```python
from build123d import *

# Parameters (mm, degrees)
ESQUISSE1_W        = 94
ESQUISSE1_H        = 61
ESQUISSE1_R        = 1.75
BOSS_EXTRU_1_DEPTH = 1.6
ESQUISSE2_W        = 50
ESQUISSE2_H        = 25
BOSS_EXTRU_2_DEPTH = 18
ESQUISSE3_W        = 9
ESQUISSE3_H        = 14
BOSS_EXTRU_3_DEPTH = 11


with BuildPart() as part:
    # Esquisse1 → Boss.-Extru.1 (new body)
    with BuildSketch(Plane.XY):
        Rectangle(ESQUISSE1_W, ESQUISSE1_H)
        with Locations((-42, 25.5)):
            Circle(ESQUISSE1_R, mode=Mode.SUBTRACT)
        with Locations((42, 25.5)):
            Circle(ESQUISSE1_R, mode=Mode.SUBTRACT)
        with Locations((42, -25.5)):
            Circle(ESQUISSE1_R, mode=Mode.SUBTRACT)
        with Locations((-42, -25.5)):
            Circle(ESQUISSE1_R, mode=Mode.SUBTRACT)
    extrude(amount=BOSS_EXTRU_1_DEPTH)

    # Esquisse2 → Boss.-Extru.2 (add)
    with BuildSketch(Plane.XY.offset(1.6)):
        Rectangle(ESQUISSE2_W, ESQUISSE2_H)
    extrude(amount=BOSS_EXTRU_2_DEPTH)

    # Esquisse3 → Boss.-Extru.3 (add)
    with BuildSketch(Plane.XY.offset(1.6)):
        with Locations((-31.5, -23.5)):
            Rectangle(ESQUISSE3_W, ESQUISSE3_H)
    extrude(amount=BOSS_EXTRU_3_DEPTH)


solid = part.part
```
Design review of the part built by this model. Coordinates are the model's own, in mm. A direction names the side the tool comes from. Give positions to 0.01 mm unless a question says otherwise; leave off trailing zeros. Write each loop counter-clockwise with the first axis right and the second up, starting at its lowest first coordinate (ties: lowest second). Pieces come first, ordered by that corner, then holes. Notation, with made-up numbers: (0.25, 89) -> (14.25, 89) arc R7 ccw to (14.25, 96) -> close; hole circle Ø9 at (65, 44.5). An arc over 180 degrees is marked (long way). Answer in a Markdown table with one row per item.
(1) Consider section A-A (x = 42). State the section outline as (y, z) points.
Results:
| item | result |
|---|---|
| outline | (-30.5, 0) -> (-27.25, 0) -> (-27.25, 1.6) -> (-30.5, 1.6) -> close; (-23.75, 0) -> (23.75, 0) -> (23.75, 1.6) -> (-23.75, 1.6) -> close; (27.25, 0) -> (30.5, 0) -> (30.5, 1.6) -> (27.25, 1.6) -> close |
(2) Consider section C-C (y = -25.5). State the section outline as (x, z) points.
Results:
| item | result |
|---|---|
| outline | (-47, 0) -> (-43.75, 0) -> (-43.75, 1.6) -> (-47, 1.6) -> close; (-40.25, 0) -> (40.25, 0) -> (40.25, 1.6) -> (-27, 1.6) -> (-27, 12.6) -> (-36, 12.6) -> (-36, 1.6) -> (-40.25, 1.6) -> close; (43.75, 0) -> (47, 0) -> (47, 1.6) -> (43.75, 1.6) -> close |
(3) For faces 4 (the flat face through (-25, 0, 10)), 5 (the flat face through (25, 0, 10)), 6 (the flat face through (0, 12.5, 10)), list the 3-axis set-ups (+Z, -Z, +X, -X, +Y, -Y) from which the entire face can be reached by the end or side of a thin tool; tool diameter is ignored.
Results:
| item | result |
|---|---|
| face 4 | +Z, -X, +Y, -Y |
| face 5 | +Z, +X, +Y, -Y |
| face 6 | +Z, +X, -X, +Y |
(4) Mouldability with a two-part tool opening along Y and no side actions: class faces 1 (the cylindrical face through (-41.1, -24, 0.8)), 2 (the flat face through (0, -12.5, 10)), 3 (the flat face through (-27, -24, 7)) as +Y half, -Y half, draft (parallel to the pull), parting line (faces both ways), or undercut.
Results:
| item | result |
|---|---|
| face 1 | undercut |
| face 2 | -Y half |
| face 3 | draft |
(5) To check wall thickness, follow probe 1 along Y at (x, z) = (42, 0.8); probe 2 along Y at (x, z) = (-24, 15); probe 3 along Z at (x, y) = (-9.5, 23.5). State the ranges of each line that lie inside material, in increasing order.
Results:
| item | result |
|---|---|
| probe 1 | -30.5 to -27.25, -23.75 to 23.75, 27.25 to 30.5 |
| probe 2 | -12.5 to 12.5 |
| probe 3 | 0 to 1.6 |
(6) Consider section B-B (z = 5.5). State the section outline as (x, y) points.
Results:
| item | result |
|---|---|
| outline | (-36, -30.5) -> (-27, -30.5) -> (-27, -16.5) -> (-36, -16.5) -> close; (-25, -12.5) -> (25, -12.5) -> (25, 12.5) -> (-25, 12.5) -> close |
(7) Clearance check with flat-ended pins moving along their axes: pin 1 (1 mm diameter, centred on x = 10, z = 2.5, fed in from -Y); pin 2 (5.5 mm diameter, centred on y = -22.5, z = 8.5, fed in from +X); pin 3 (4.5 mm diameter, centred on x = -33.5, z = 9.5, fed in from +Y); pin 4 (2 mm diameter, centred on x = 42, y = -25.5, fed in from -Z). State where each tip first meets the part, or that it passes through.
Results:
| item | result |
|---|---|
| pin 1 | y = -12.5 |
| pin 2 | x = -27 |
| pin 3 | y = -16.5 |
| pin 4 | through |
(8) Consider section D-D (y = 3). State the section outline as (x, z) points.
Results:
| item | result |
|---|---|
| outline | (-47, 0) -> (47, 0) -> (47, 1.6) -> (25, 1.6) -> (25, 19.6) -> (-25, 19.6) -> (-25, 1.6) -> (-47, 1.6) -> close |
